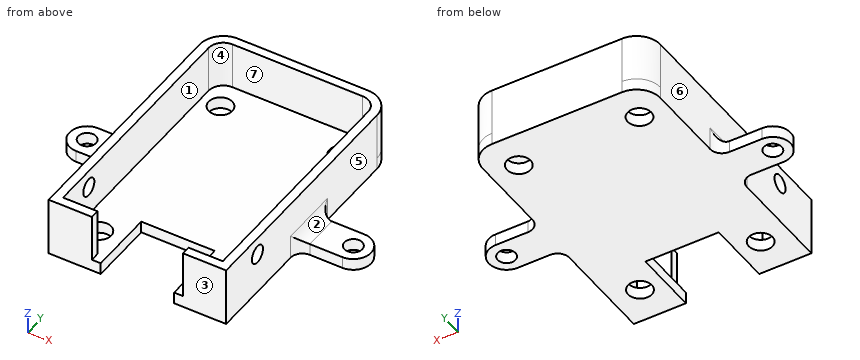
```python
from build123d import *

# Parameters (mm, degrees)
ESQUISSE1_W                  = 30
ESQUISSE1_H                  = 45
BOSS_EXTRU_1_DEPTH           = 2
ESQUISSE3_R                  = 2
ESQUISSE3_W                  = 12.4
ESQUISSE3_H                  = 11
ENL_V_MAT_EXTRU_1_DEPTH      = 28.115494
CONG_1_R                     = 4
BOSS_EXTRU_2_START           = 10
BOSS_EXTRU_2_DEPTH           = 10
ENL_V_MAT_EXTRU_2_DEPTH      = 29.831406
ENL_V_MAT_EXTRU_2_DEPTH_BACK = 29.831406
ESQUISSE7_R                  = 1.5
ESQUISSE10_R                 = 1.5
BOSS_EXTRU_3_DEPTH           = 2
CONG_2_R                     = 2
CONG_3_R                     = 2


with BuildPart() as part:
    # Esquisse1 → Boss.-Extru.1 (new body)
    with BuildSketch(Plane.XY):
        Rectangle(ESQUISSE1_W, ESQUISSE1_H)
    extrude(amount=BOSS_EXTRU_1_DEPTH)

    # Esquisse3 → Enlèv. mat.-Extru.1 (cut, through all)
    with BuildSketch(Plane.XY):
        with Locations((10.2, 16.45)):
            Circle(ESQUISSE3_R)
        with Locations(Location((-10.2, 16.45, 0), (0, 0, 180))):
            Circle(ESQUISSE3_R)
        with Locations((-10.2, -16.45)):
            Circle(ESQUISSE3_R)
        with Locations(Location((10.2, -16.45, 0), (0, 0, 180))):
            Circle(ESQUISSE3_R)
        with Locations((0, -17)):
            Rectangle(ESQUISSE3_W, ESQUISSE3_H)
    extrude(amount=ENL_V_MAT_EXTRU_1_DEPTH, mode=Mode.SUBTRACT)

    # Congé1
    cong_1_edges = [part.edges().sort_by_distance(p)[0] for p in [
        (-15, 22.5, 1),
        (15, 22.5, 1),
    ]]
    fillet(cong_1_edges, radius=CONG_1_R)

    # Esquisse6 → Boss.-Extru.2 (add)
    with BuildSketch(Plane.XY.offset(BOSS_EXTRU_2_START)):
        with BuildLine():
            Line((7.7, -21), (7.7, -22.5))
            Line((7.7, -22.5), (15, -22.5))
            Line((15, -22.5), (15, 18.5))
            ThreePointArc((15, 18.5), (13.828427, 21.328427), (11, 22.5))
            Line((11, 22.5), (-11, 22.5))
            ThreePointArc((-11, 22.5), (-13.828427, 21.328427), (-15, 18.5))
            Line((-15, 18.5), (-15, -22.5))
            Line((-15, -22.5), (-7.7, -22.5))
            Line((-7.7, -22.5), (-7.7, -21))
            Line((-7.7, -21), (-13.5, -21))
            Line((-13.5, -21), (-13.5, 18.5))
            ThreePointArc((-13.5, 18.5), (-12.767767, 20.267767), (-11, 21))
            Line((-11, 21), (11, 21))
            ThreePointArc((11, 21), (12.767767, 20.267767), (13.5, 18.5))
            Line((13.5, 18.5), (13.5, -21))
            Line((13.5, -21), (7.7, -21))
        make_face()
    extrude(amount=-BOSS_EXTRU_2_DEPTH)

    # Esquisse7 → Enlèv. mat.-Extru.2 (cut, two sides: drawn at the far end of the back side and taken through both)
    with BuildSketch(Plane(origin=(0, 0, 0), x_dir=(0, 0, -1), z_dir=(1, 0, 0)).offset(-ENL_V_MAT_EXTRU_2_DEPTH_BACK)):
        with Locations((-7, -14)):
            Circle(ESQUISSE7_R)
    extrude(amount=ENL_V_MAT_EXTRU_2_DEPTH + ENL_V_MAT_EXTRU_2_DEPTH_BACK, mode=Mode.SUBTRACT)

    # Esquisse10 → Boss.-Extru.3 (add)
    with BuildSketch(Plane.XY):
        with BuildLine():
            Line((15, 3), (22.5, 3))
            ThreePointArc((22.5, 3), (25.5, 0), (22.5, -3))
            Line((22.5, -3), (15, -3))
            Line((15, -3), (15, 3))
        make_face()
        with Locations((22.5, 0)):
            Circle(ESQUISSE10_R, mode=Mode.SUBTRACT)
    boss_extru_3 = extrude(amount=BOSS_EXTRU_3_DEPTH)

    # Congé2
    cong_2_edges = [part.edges().sort_by_distance(p)[0] for p in [
        (15, 0, 2),
        (15, 3, 1),
        (15, -3, 1),
    ]]
    fillet(cong_2_edges, radius=CONG_2_R)

    # Symétrie2: Boss.-Extru.3 across plane
    add(boss_extru_3.mirror(Plane(origin=(0, 0, 0), x_dir=(0, 0, 1), z_dir=(1, 0, 0))))

    # Congé3
    cong_3_edges = [part.edges().sort_by_distance(p)[0] for p in [
        (-15, 0, 2),
        (-15, -3, 1),
        (-15, 3, 1),
    ]]
    fillet(cong_3_edges, radius=CONG_3_R)


solid = part.part
```
Here's how the part is built. I have some questions about the finished solid (model axes, mm). Face numbers are marked on the shaded views. A direction names the side the tool comes from. Give positions to 0.01 mm unless a question says otherwise; leave off trailing zeros. Write each loop counter-clockwise with the first axis right and the second up, starting at its lowest first coordinate (ties: lowest second). Pieces come first, ordered by that corner, then holes. Notation, with made-up numbers: M 53,-19.5 L 63,-19.5 A14 cw 63,7.5 Z; hole C 22.25,20.5 d6. An arc over 180 degrees is marked long. Put each result on its own line as item: value. Start each with the question number.
Item 1: Thinking about a two-plate mould opening in Y: for the marked faces 1, 2, 3 and 4, which applies, +Y half, -Y half, draft (parallel to the pull), parting line (faces both ways), or undercut?
Item 2: On a 3-axis mill with a long thin cutter (end or side, diameter ignored), from which of +Z, -Z, +X, -X, +Y, -Y can I reach the whole of each face in a straight line? I mean the marked faces 5, 6 and 7. Say none if no direction works.
Item 3: Will these pins go through, and if not, where does the flat tip stop? pin 1 (6.5 mm diameter, centred on x = 19.5, y = -1.5, fed in from +Z); pin 2 (1.8 mm diameter, centred on x = -19.5, y = 0, fed in from +Z); pin 3 (2 mm diameter, centred on y = 4.5, z = 4, fed in from +X).
Item 4: If we section it at B-B, the plane z = 7: Write out the boundary of the cut face in (x, y).
Item 5: If we section it at A-A, the plane y = -16.45: Write out the boundary of the cut face in (x, z).
Item 6: If we section it at C-C, the plane x = 10.2: Write out the boundary of the cut face in (y, z), then the cut area to 3 significant figures.
Item 7: I need wall thicknesses on L1, parallel to Y at x = 10.2, z = 0.95; L2, parallel to X at y = -16.45, z = 1.3; L3, parallel to X at y = 16.45, z = 0.7. Which ranges of each line are inside material? Lowest first, please. Write a range as from..to.
Item 8: If we section it at D-D, the plane y = 0: Write out the boundary of the cut face in (x, z).
Values:
1. face 1: undercut
1. face 2: draft
1. face 3: -Y half
1. face 4: undercut
2. face 5: +Z, +X
2. face 6: +Z, -X
2. face 7: +Z
3. pin 1: z = 2.15
3. pin 2: z = 2
3. pin 3: x = 15.22
4. outline: M -15,-22.5 L -7.7,-22.5 L -7.7,-21 L -13.5,-21 L -13.5,-15.5 L -15,-15.5 Z; M -15,-12.5 L -13.5,-12.5 L -13.5,18.5 A2.5 cw -11,21 L 11,21 A2.5 cw 13.5,18.5 L 13.5,-12.5 L 15,-12.5 L 15,18.5 A4 ccw 11,22.5 L -11,22.5 A4 ccw -15,18.5 Z; M 7.7,-22.5 L 15,-22.5 L 15,-15.5 L 13.5,-15.5 L 13.5,-21 L 7.7,-21 Z
5. outline: M -15,0 L -12.2,0 L -12.2,2 L -13.5,2 L -13.5,10 L -15,10 Z; M -8.2,0 L -6.2,0 L -6.2,2 L -8.2,2 Z; M 6.2,0 L 8.2,0 L 8.2,2 L 6.2,2 Z; M 12.2,0 L 15,0 L 15,10 L 13.5,10 L 13.5,2 L 12.2,2 Z
6. outline: M -22.5,0 L -18.45,0 L -18.45,2 L -21,2 L -21,10 L -22.5,10 Z; M -14.45,0 L 14.45,0 L 14.45,2 L -14.45,2 Z; M 18.45,0 L 22.5,0 L 22.5,10 L 21,10 L 21,2 L 18.45,2 Z
6. area: 98.0 mm²
7. L1: -22.5..-18.45, -14.45..14.45, 18.45..22.5
7. L2: -15..-12.2, -8.2..-6.2, 6.2..8.2, 12.2..15
7. L3: -15..-12.2, -8.2..8.2, 12.2..15
8. outline: M -25.5,0 L -24,0 L -24,2 L -25.5,2 Z; M -21,0 L 21,0 L 21,2 L 17,2 A2 cw 15,4 L 15,10 L 13.5,10 L 13.5,2 L -13.5,2 L -13.5,10 L -15,10 L -15,4 A2 cw -17,2 L -21,2 Z; M 24,0 L 25.5,0 L 25.5,2 L 24,2 Z
